```python
from build123d import *

# Parameters (mm, degrees)
F0_W     = 11
F0_H     = 26
F1_DEPTH = 3
F2_W     = 11
F2_H     = 12
F3_DEPTH = 1
F5_D     = 2.1


with BuildPart() as f1:
    # F0 (on Top) → F1 (new body)
    with BuildSketch(Plane.XY):
        Rectangle(F0_W, F0_H)
    extrude(amount=F1_DEPTH)

    # F2 (on face) → F3 (cut)
    with BuildSketch(Plane(origin=(0, 0, 0), x_dir=(1, 0, 0), z_dir=(0, 0, -1))):
        Rectangle(F2_W, F2_H)
    extrude(amount=-F3_DEPTH, mode=Mode.SUBTRACT)

    # F5 (through all)
    with Locations(Plane.XY.offset(3)):
        with Locations((0, 10), (0, -10)):
            Hole(F5_D / 2)


solid = f1.part
```
CAD build for the part. Positions are in the model's coordinates, mm. A direction names the side the tool comes from. Coordinates: 2 decimals unless noted, no trailing zeros. Loops run counter-clockwise (first coordinate to the right, second up) from the corner with the lowest first, then second, coordinate; pieces in that order, holes last. Notation, with made-up numbers: (54, -1.5) - (89, -1.5) arc R24 cw to (89, 34.5) - close; hole circle Ø6 at (-23.75, -7). An arc over 180 degrees is marked (long way). Return JSON: item names as keys, results as strings.
1. Probe L1, parallel to Y at x = 0, z = 1.4; L2, parallel to Y at x = 0, z = 0.8; L3, parallel to Y at x = -3.75, z = 0.4. List the from-to ranges inside material, lowest first. Write a range as from..to.
Result:
{"L1": "y = -13..-11.05, -8.95..8.95, 11.05..13", "L2": "y = -13..-11.05, -8.95..-6, 6..8.95, 11.05..13", "L3": "y = -13..-6, 6..13"}
2. Mould opens along X. For faces 3 (the cylindrical face through (-0.56, 10.89, 1.48)), 4 (the flat face through (-5.5, 0, 2)), 5 (the flat face through (0, -13, 1)) say: released by +X, released by -X, zero draft, split by the parting line, or undercut.
Result:
{"face 3": "undercut", "face 4": "released by -X", "face 5": "zero draft"}
3. Band-saw the part on A-A (x = 0). Give the cut face in (y, z).
Result:
{"outline": "(-13, 0) - (-11.05, 0) - (-11.05, 3) - (-13, 3) - close; (-8.95, 0) - (-6, 0) - (-6, 1) - (6, 1) - (6, 0) - (8.95, 0) - (8.95, 3) - (-8.95, 3) - close; (11.05, 0) - (13, 0) - (13, 3) - (11.05, 3) - close"}
4. Band-saw the part on B-B (y = -10). Give the cut face in (x, z), and give its area (3 significant figures).
Result:
{"outline": "(-5.5, 0) - (-1.05, 0) - (-1.05, 3) - (-5.5, 3) - close; (1.05, 0) - (5.5, 0) - (5.5, 3) - (1.05, 3) - close", "area": "26.7 mm2"}
5. Band-saw the part on D-D (x = 2). Give the cut face in (y, z), and give its area (3 significant figures).
Result:
{"outline": "(-13, 0) - (-6, 0) - (-6, 1) - (6, 1) - (6, 0) - (13, 0) - (13, 3) - (-13, 3) - close", "area": "66.0 mm2"}
6. Band-saw the part on C-C (z = 2.35). Give the cut face in (x, y), and give its area (3 significant figures).
Result:
{"outline": "(-5.5, -13) - (5.5, -13) - (5.5, 13) - (-5.5, 13) - close; hole circle Ø2.1 at (0, -10); hole circle Ø2.1 at (0, 10)", "area": "279 mm2"}
7. Drop a flat-ended pin along its axis: pin 1 (5.5 mm diameter, centred on x = -2.5, y = -2, fed in from -Z). Give the stop position or say it passes through.
Result:
{"pin 1": "stops at z = 1"}
8. 3-axis set-ups, long thin cutter, end or side, ignore diameter. For faces 1 (the flat face through (-0.1, 6, 0.5)), 2 (the flat face through (-0.1, -8.7, 0)): which of +Z, -Z, +X, -X, +Y, -Y reach the whole face in a straight line?
Result:
{"face 1": "-Z, +X, -X", "face 2": "-Z, +X, -X, +Y, -Y"}
